Could you check a few things on this drawing? It's one solid part, dimensions in mm from its lowest x, y, z. A direction names the side the tool comes from. Give positions to 0.01 mm unless a question says otherwise; leave off trailing zeros. Loops run counter-clockwise (first coordinate to the right, second up) from the corner with the lowest first, then second, coordinate; pieces in that order, holes last. Notation, with made-up numbers: (-3, 38) - (16, 38) arc R27 ccw to (16, 75) - close; hole circle Ø9 at (87, 3.25). An arc over 180 degrees is marked (long way). Write item = value, one per line.
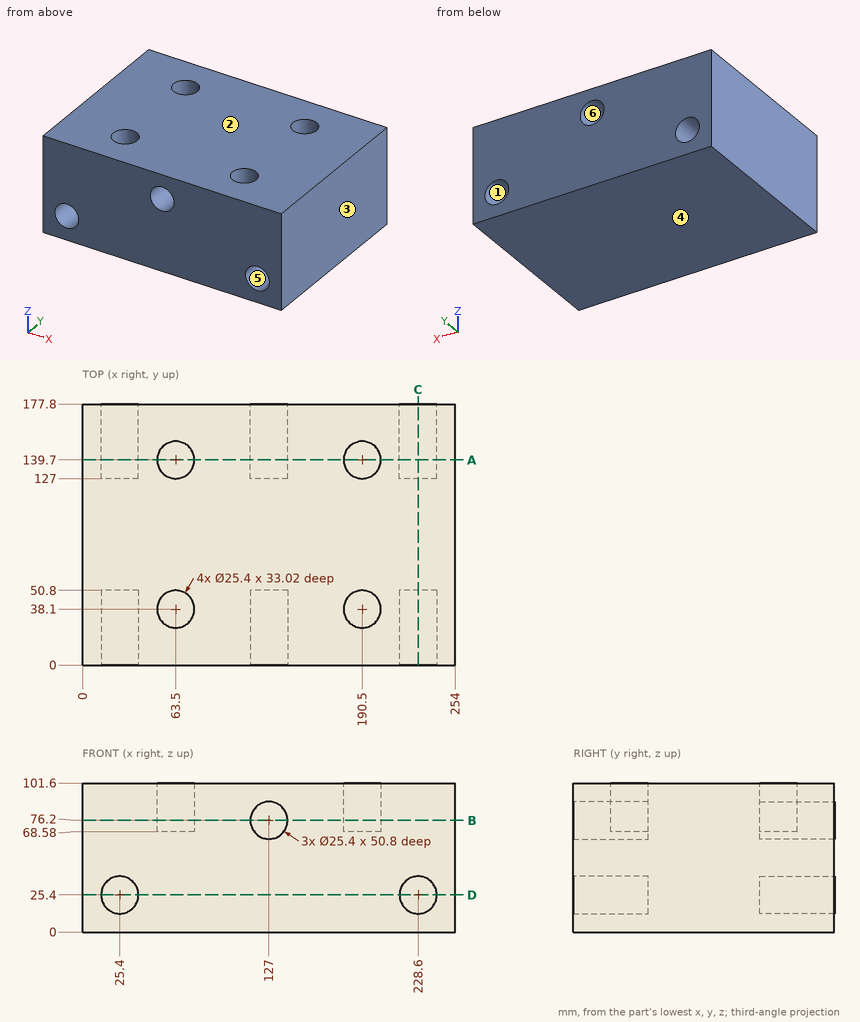
Q1. Imagine slicing it at B-B, the plane z = 76.2. Write out the boundary of the cut face in (x, y).
Output:
outline = (0, 0) - (114.3, 0) - (114.3, 50.8) - (139.7, 50.8) - (139.7, 0) - (254, 0) - (254, 177.8) - (139.7, 177.8) - (139.7, 127) - (114.3, 127) - (114.3, 177.8) - (0, 177.8) - close; hole circle Ø25.4 at (63.5, 38.1); hole circle Ø25.4 at (63.5, 139.7); hole circle Ø25.4 at (190.5, 38.1); hole circle Ø25.4 at (190.5, 139.7)
Q2. We'd pull the mould along Z, two halves only. Please class the marked faces 1, 2 and 3: released by +Z, released by -Z, zero draft, split by the parting line, or undercut.
Output:
face_1 = undercut
face_2 = released by +Z
face_3 = zero draft
Q3. I need wall thicknesses on L1, parallel to X at y = 33.5, z = 25.4; L2, parallel to Y at x = 190.5, z = 92.5; L3, parallel to X at y = 139, z = 83. Which ranges of each line are inside material? Lowest first, please.
Output:
L1 = 0 to 12.7, 38.1 to 215.9, 241.3 to 254
L2 = 0 to 25.4, 50.8 to 127, 152.4 to 177.8
L3 = 0 to 50.82, 76.18 to 116.27, 137.73 to 177.82, 203.18 to 254
Q4. For pin 1 (15 mm diameter, centred on x = 228.6, z = 25.4, fed in from +Y); pin 2 (7.5 mm diameter, centred on x = 63, y = 143.5, fed in from +Z); pin 3 (15 mm diameter, centred on x = 127, z = 76.2, fed in from -Y), each with a flat end and sliding along its axis, tell me the tip position at first contact or that it passes through.
Output:
pin_1 = 127
pin_2 = 68.58
pin_3 = 50.8
Q5. Imagine slicing it at A-A, the plane y = 139.7. Write out the boundary of the cut face in (x, z), then the cut area to 3 significant figures.
Output:
outline = (0, 0) - (254, 0) - (254, 101.6) - (203.2, 101.6) - (203.2, 68.58) - (177.8, 68.58) - (177.8, 101.6) - (76.2, 101.6) - (76.2, 68.58) - (50.8, 68.58) - (50.8, 101.6) - (0, 101.6) - close; hole circle Ø25.4 at (25.4, 25.4); hole circle Ø25.4 at (127, 76.2); hole circle Ø25.4 at (228.6, 25.4)
area = 22,600 mm2
Q6. Imagine slicing it at D-D, the plane z = 25.4. Write out the boundary of the cut face in (x, y), then the cut area to 3 significant figures.
Output:
outline = (0, 0) - (12.7, 0) - (12.7, 50.8) - (38.1, 50.8) - (38.1, 0) - (215.9, 0) - (215.9, 50.8) - (241.3, 50.8) - (241.3, 0) - (254, 0) - (254, 177.8) - (241.3, 177.8) - (241.3, 127) - (215.9, 127) - (215.9, 177.8) - (38.1, 177.8) - (38.1, 127) - (12.7, 127) - (12.7, 177.8) - (0, 177.8) - close
area = 40,000 mm2
Q7. Which directions (+Z, -Z, +X, -X, +Y, -Y) give clear straight access to the entire face, cutting with the end or side of a thin tool? Please do the marked faces 4, 5 and 6.
Output:
face_4 = -Z, +X, -X, +Y, -Y
face_5 = -Y
face_6 = +Y
Q8. Imagine slicing it at C-C, the plane x = 228.6. Write out the boundary of the cut face in (y, z), then the cut area to 3 significant figures.
Output:
outline = (0, 0) - (177.8, 0) - (177.8, 12.7) - (127, 12.7) - (127, 38.1) - (177.8, 38.1) - (177.8, 101.6) - (0, 101.6) - (0, 38.1) - (50.8, 38.1) - (50.8, 12.7) - (0, 12.7) - close
area = 15,500 mm2
